Design review of the part built by this model. Coordinates are the model's own, in mm. Face numbers are marked on the shaded views. Coordinates: 2 decimals unless noted, no trailing zeros. Write each loop counter-clockwise with the first axis right and the second up, starting at its lowest first coordinate (ties: lowest second). Pieces come first, ordered by that corner, then holes.
Autodesk Inventor part; units mm, degrees
ref_plane "YZ Plane" through (0, 0, 0) normal (1, 0, 0) x (0, 1, 0)
ref_plane "XZ Plane" through (0, 0, 0) normal (0, 1, 0) x (-1, 0, 0)
ref_plane "XY Plane" through (0, 0, 0) normal (0, 0, 1) x (1, 0, 0)
sketch "Sketch1" plane through (0, 0, 0) normal (0, 1, 0) x (-1, 0, 0)
  line L0 (-33.5, 8) -> (33.5, 8)
  line L1 (33.5, 8) -> (33.5, -8)
  line L2 (33.5, -8) -> (-33.5, -8)
  line L3 (-33.5, -8) -> (-33.5, 8)
  line L4 (-33.5, 8) -> (33.5, -8) construction
  line L5 (33.5, 8) -> (-33.5, -8) construction
  line L6 (46.9, 0) -> (-46.9, 0) construction
  line L7 (0, -11.2) -> (0, 11.2) construction
  line L8 (26, 0) -> (-26, 0)
  circle A0 centre (26, 0) radius 3.75
  circle A1 centre (-26, 0) radius 3.75
  point P0 (0, 0)
  dimension "d0" = 16
  dimension "d1" = 67
  dimension "d2" = 52
  dimension "d3" = 7.5
extrude "Extrusion1" add sketch "Sketch1" along normal blind 8
fillet "Fillet1" radius 2 4 edges at (33.5, 4, 8) (-33.5, 4, 8) (-33.5, 4, -8) (33.5, 4, -8)
properties part number "07_Mieng_go_bu_67x16" material "Laminated Veneer Lumber"
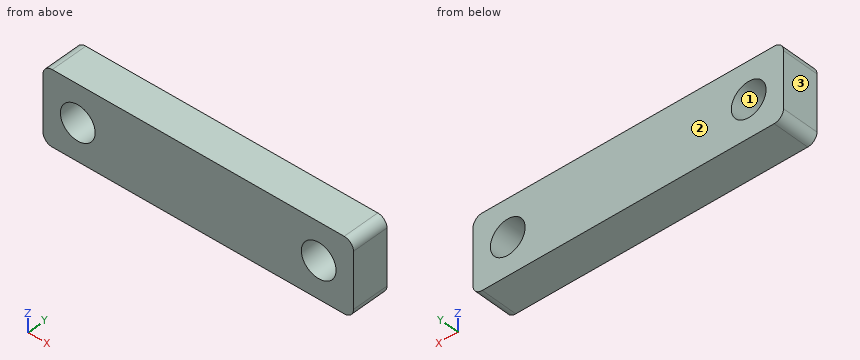
(1) Wall thickness on line 1 (X direction, y = 0.5, z = -0.25); line 2 (Z direction, x = 26, y = 6); line 3 (Z direction, x = 23, y = 2.5): over which ranges is each line inside the solid? List them lowest first.
(2) Mouldability with a two-part tool opening along X and no side actions: class the marked faces 1, 2 and 3 as +X half, -X half, draft (parallel to the pull), parting line (faces both ways), or undercut.
(3) Consider section A-A (x = -26). Give the boundary of the cut face in (y, z).
(4) Consider section B-B (z = 0). Give the boundary of the cut face in (x, y), plus the area to 3 significant figures.
(5) Consider section D-D (z = 2.75). Give the boundary of the cut face in (x, y).
(6) Insertion check: pin 1 Ø7 at (x, z) = (-26, 0) entering from +Y. The pin has a flat end and moves straight along its axis. Give the tip position at first contact, or say it passes through.
(7) Consider section C-C (y = 6). Give the boundary of the cut face in (x, z), plus the area to 3 significant figures.
Results:
1. line 1: x = -33.5 to -29.74, -22.26 to 22.26, 29.74 to 33.5
1. line 2: z = -8 to -3.75, 3.75 to 8
1. line 3: z = -8 to -2.25, 2.25 to 8
2. face 1: undercut
2. face 2: draft
2. face 3: -X half
3. outline: (0, -8) - (8, -8) - (8, -3.75) - (0, -3.75) - close; (0, 3.75) - (8, 3.75) - (8, 8) - (0, 8) - close
4. outline: (-33.5, 0) - (-29.75, 0) - (-29.75, 8) - (-33.5, 8) - close; (-22.25, 0) - (22.25, 0) - (22.25, 8) - (-22.25, 8) - close; (29.75, 0) - (33.5, 0) - (33.5, 8) - (29.75, 8) - close
4. area: 416 mm2
5. outline: (-33.5, 0) - (-28.55, 0) - (-28.55, 8) - (-33.5, 8) - close; (-23.45, 0) - (23.45, 0) - (23.45, 8) - (-23.45, 8) - close; (28.55, 0) - (33.5, 0) - (33.5, 8) - (28.55, 8) - close
6. pin 1: passes through
7. outline: (-33.5, -6) arc R2 ccw to (-31.5, -8) - (31.5, -8) arc R2 ccw to (33.5, -6) - (33.5, 6) arc R2 ccw to (31.5, 8) - (-31.5, 8) arc R2 ccw to (-33.5, 6) - close; hole circle Ø7.5 at (-26, 0); hole circle Ø7.5 at (26, 0)
7. area: 980 mm2
